The model under review builds one solid part; all positions refer to its coordinate system, in mm. A direction names the side the tool comes from. Give positions to 0.01 mm unless a question says otherwise; leave off trailing zeros. Order: outer loops, then holes, each group sorted by start corner. A loop starts at its lowest first (then second) coordinate and runs counter-clockwise, first axis right, second up. Notation, with made-up numbers: (6, 1.25) - (17, 1.25) arc R4 ccw to (17, 8.25) - close; hole circle Ø9 at (25, -38.75). An arc over 180 degrees is marked (long way). Write item = value, one per line. Start each with the question number.
1. We need section B-B, the plane y = 4.75. Give the boundary of the cut face in (x, z), and give its area (3 significant figures).
2. Wall thickness on probe 1 along Z at (x, y) = (0, 5.25); probe 2 along X at (y, z) = (2.25, -12.7); probe 3 along Z at (x, y) = (1.5, 1.5): over which ranges is each line inside the solid? List them lowest first.
3. We need section C-C, the plane x = 50.8. Give the boundary of the cut face in (y, z).
4. We need section D-D, the plane z = 12.7. Give the boundary of the cut face in (x, y), and give its area (3 significant figures).
5. We need section A-A, the plane x = 0. Give the boundary of the cut face in (y, z), and give its area (3 significant figures).
6. For P1, Ø5, axis at x = 0, z = 0, coming from the +Y side; P2, Ø3, axis at x = 38.1, z = -12.7, coming from the -Y side; P3, Ø1.9, axis at x = 46, y = 2, coming from the +Z side, all flat-tipped, find the tip position at first contact; note any pin that passes through.
7. Mouldability with a two-part tool opening along X and no side actions: class faces 1 (the cylindrical face through (-11.707, 3.219, -24.458)), 2 (the flat face through (36, 3, 0)), 3 (the cylindrical face through (13.642, 3.131, 0.993)), 4 (the cylindrical face through (-0.6, 3.13, 14.59)) as pulls with the +X half, pulls with the -X half, needs draft (parallel to the pull), parting line crosses it, or undercut.
8. Machinability: for faces 5 (the flat face through (0, 3, 25.4)), 6 (the flat face through (12.7, 3, 15)), which of the approach directions +Z, -Z, +X, -X, +Y, -Y give a long, thin tool a straight path to every point of the face, cutting with its end or side? Answer none if there is none.
Autodesk Inventor part; units mm, degrees
ref_plane "YZ Plane" through (0, 0, 0) normal (1, 0, 0) x (0, 1, 0)
ref_plane "XZ Plane" through (0, 0, 0) normal (0, 1, 0) x (-1, 0, 0)
ref_plane "XY Plane" through (0, 0, 0) normal (0, 0, 1) x (1, 0, 0)
sketch "Sketch1" plane through (0, 0, 0) normal (0, 1, 0) x (-1, 0, 0)
  line L0 (12.7, 25.4) -> (-12.7, 25.4)
  line L1 (-12.7, 25.4) -> (-12.7, -25.4)
  line L2 (-12.7, -25.4) -> (12.7, -25.4)
  line L3 (12.7, -25.4) -> (12.7, 25.4)
  line L4 (12.7, 25.4) -> (-12.7, -25.4) construction
  line L5 (-12.7, 25.4) -> (12.7, -25.4) construction
  point P0 (0, 0)
  dimension "d0" = 25.4
  dimension "d1" = 50.8
extrude "Extrusion1" add sketch "Sketch1" along normal blind 6.35
sketch "Sketch3" plane through (12.7, 0, 25.4) normal (1, 0, 0) x (0, 0, -1)
  line L0 (0, 6.35) -> (50.8, 6.35)
  line L1 (50.8, 6.35) -> (25.4, 6.35)
  line L2 (25.4, 6.35) -> (25.4, 0)
  line L3 (25.4, 0) -> (50.8, 0)
  line L4 (50.8, 0) -> (50.8, 6.35)
  dimension "d14" = 25.4
extrude "Extrusion2" add sketch "Sketch3" along normal blind 44.45
sketch "Sketch4" plane through (0, 6.35, 0) normal (0, 1, 0) x (1, 0, 0)
  line L0 (-12.7, -25.4) -> (12.7, -25.4)
  point P0 (0, 0)
  point P1 (0, -12.7)
  point P2 (0, 0)
  point P3 (0, 12.7)
  point P4 (0, -25.4)
  point P5 (0, -25.4)
  point P6 (0, -25.4)
  point P7 (25.4, 12.7)
  point P8 (38.1, 12.7)
  point P9 (50.8, 12.7)
  dimension "d17" = 12.7
  dimension "d18" = 12.7
  dimension "d19" = 12.7
  dimension "d20" = 25.4
  dimension "d21" = 12.7
  dimension "d22" = 12.7
hole "Hole2" at (0, 6.35, 12.7) at (0, 6.35, 0) at (0, 6.35, -12.7) at (25.4, 6.35, -12.7) at (38.1, 6.35, -12.7) at (50.8, 6.35, -12.7) direction (0, -1, 0) diameter 3.9624 end through all
fillet "Fillet1" radius 3.302 2 edges at (12.7, 3.175, 0) (-12.7, 3.175, -25.4)
properties part number "DB1-004" material "Aluminum 6061"
Model answer:
q1.outline = (-12.7, -22.1) arc R3.3 ccw to (-9.4, -25.4) - (57.15, -25.4) - (57.15, 0) - (16, 0) arc R3.3 cw to (12.7, 3.3) - (12.7, 25.4) - (-12.7, 25.4) - close; hole circle Ø3.96 at (0, -12.7); hole circle Ø3.96 at (0, 0); hole circle Ø3.96 at (0, 12.7); hole circle Ø3.96 at (25.4, -12.7); hole circle Ø3.96 at (38.1, -12.7); hole circle Ø3.96 at (50.8, -12.7)
q1.area = 2,350 mm2
q2.probe_1 = -25.4 to -14.68, -10.72 to -1.98, 1.98 to 10.72, 14.68 to 25.4
q2.probe_2 = -12.7 to -1.98, 1.98 to 23.42, 27.38 to 36.12, 40.08 to 48.82, 52.78 to 57.15
q2.probe_3 = -25.4 to -13.99, -11.41 to -1.29, 1.29 to 11.41, 13.99 to 25.4
q3.outline = (0, -25.4) - (6.35, -25.4) - (6.35, -14.68) - (0, -14.68) - close; (0, -10.72) - (6.35, -10.72) - (6.35, 0) - (0, 0) - close
q4.outline = (-12.7, 0) - (-1.98, 0) - (-1.98, 6.35) - (-12.7, 6.35) - close; (1.98, 0) - (12.7, 0) - (12.7, 6.35) - (1.98, 6.35) - close
q4.area = 136 mm2
q5.outline = (0, -25.4) - (6.35, -25.4) - (6.35, -14.68) - (0, -14.68) - close; (0, -10.72) - (6.35, -10.72) - (6.35, -1.98) - (0, -1.98) - close; (0, 1.98) - (6.35, 1.98) - (6.35, 10.72) - (0, 10.72) - close; (0, 14.68) - (6.35, 14.68) - (6.35, 25.4) - (0, 25.4) - close
q5.area = 247 mm2
q6.P1 = 6.35
q6.P2 = through
q6.P3 = 0
q7.face_1 = pulls with the -X half
q7.face_2 = needs draft
q7.face_3 = pulls with the +X half
q7.face_4 = undercut
q8.face_5 = +Z, +X, -X, +Y, -Y
q8.face_6 = +Z, +X, +Y, -Y
